```python
from build123d import *

# Parameters (mm, degrees)
F1_DEPTH = 135.89


with BuildPart() as f1:
    # F0 (on Front) → F1 (new body)
    with BuildSketch(Plane.XZ):
        with BuildLine():
            ThreePointArc((-0.402361, -59.350092), (-14.92337, -57.568817), (-28.607244, -52.393469))
            ThreePointArc((-28.607244, -52.393469), (-56.848471, -62.044811), (-86.337414, -57.449427))
            ThreePointArc((-86.337414, -57.449427), (-61.850793, -119.454468), (-0.402361, -145.306161))
            ThreePointArc((-0.402361, -145.306161), (20.97924, -102.328126), (-0.402361, -59.350092))
        make_face()
        with BuildLine():
            ThreePointArc((5.353071, 26.413075), (1.351735, 13.475031), (0, 0))
            ThreePointArc((0, 0), (26.5136, -53.799627), (85.330052, -65.546792))
            ThreePointArc((85.330052, -65.546792), (121.639734, -41.326507), (135.680214, 0))
            ThreePointArc((135.680214, 0), (99.219052, 60.146836), (29.028204, 55.640959))
            ThreePointArc((29.028204, 55.640959), (15.124492, 42.700633), (5.353071, 26.413075))
        make_face()
        with BuildLine():
            ThreePointArc((-31.83483, 54.332647), (-16.674524, 42.414806), (-5.886424, 26.430855))
            ThreePointArc((-5.886424, 26.430855), (-0.266385, 26.605869), (5.353071, 26.413075))
            ThreePointArc((5.353071, 26.413075), (15.124492, 42.700633), (29.028204, 55.640959))
            ThreePointArc((29.028204, 55.640959), (-1.577442, 63.087342), (-31.83483, 54.332647))
        make_face()
        with BuildLine():
            ThreePointArc((-28.607244, -52.393469), (-7.617664, -29.84732), (0, 0))
            ThreePointArc((0, 0), (-1.489415, 13.539203), (-5.886424, 26.430855))
            ThreePointArc((-5.886424, 26.430855), (-16.674524, 42.414806), (-31.83483, 54.332647))
            ThreePointArc((-31.83483, 54.332647), (-118.264652, 27.295814), (-86.337414, -57.449427))
            ThreePointArc((-86.337414, -57.449427), (-56.848471, -62.044811), (-28.607244, -52.393469))
        make_face()
        with BuildLine():
            ThreePointArc((85.330052, -65.546792), (26.5136, -53.799627), (0, 0))
            ThreePointArc((0, 0), (-7.617664, -29.84732), (-28.607244, -52.393469))
            ThreePointArc((-28.607244, -52.393469), (-14.92337, -57.568817), (-0.402361, -59.350092))
            ThreePointArc((-0.402361, -59.350092), (20.97924, -102.328126), (-0.402361, -145.306161))
            ThreePointArc((-0.402361, -145.306161), (58.145917, -122.282952), (85.330052, -65.546792))
        make_face()
        with BuildLine():
            ThreePointArc((-5.886424, 26.430855), (-1.489415, 13.539203), (0, 0))
            ThreePointArc((0, 0), (1.351735, 13.475031), (5.353071, 26.413075))
            ThreePointArc((5.353071, 26.413075), (-0.266385, 26.605869), (-5.886424, 26.430855))
        make_face()
    extrude(amount=F1_DEPTH)


solid = f1.part
```
Work out the finished part from the listing and answer in its coordinate system (mm). Give positions to 0.01 mm unless a question says otherwise; leave off trailing zeros. Order: outer loops, then holes, each group sorted by start corner. A loop starts at its lowest first (then second) coordinate and runs counter-clockwise, first axis right, second up.
1. Each of these flat-tipped pins is pushed along its axis until it touches: P1, Ø3, axis at y = -47, z = -43.5, coming from the +X side; P2, Ø8, axis at y = -48, z = 13.5, coming from the +X side; P3, Ø1, axis at y = -113.5, z = -109.5, coming from the -X side. Where does it stop, or does it pass through?
Result sheet:
P1: stops at x = 121.12
P2: stops at x = 135.01
P3: stops at x = -70.57
2. The mould has two halves that part along X. Classify faces 1 (the cylindrical face through (-1.132, -66.994, 63.095)), 2 (the flat face through (4, 0, -14)): released by +X, released by -X, zero draft, split by the parting line, or undercut.
Result sheet:
face 1: undercut
face 2: zero draft
3. Section B-B, the plane y = -48.5 is taken. Determine the outline of the cut face in (x, z), and give its area (3 significant figures).
Result sheet:
outline: (-86.34, -57.45) arc R85.96 ccw to (85.33, -65.55) arc R67.84 ccw to (135.68, 0) arc R67.84 ccw to (29.03, 55.64) arc R61.23 ccw to (-31.83, 54.33) arc R62.28 ccw (long way) to start
area: 40,500 mm2
4. Section A-A, the plane x = -37 is taken. Determine the outline of the cut face in (y, z), and give its area (3 significant figures).
Result sheet:
outline: (-135.89, -137.13) - (0, -137.13) - (0, 56.92) - (-135.89, 56.92) - close
area: 26,400 mm2
5. Section C-C, the plane z = 40 is taken. Determine the outline of the cut face in (x, y).
Result sheet:
outline: (-110.02, -135.89) - (122.63, -135.89) - (122.63, 0) - (-110.02, 0) - close
6. Straight lines are drawn through the part: L1, parallel to Z at x = 1, y = -96; L2, parallel to X at y = -113, z = 25.5; L3, parallel to Z at x = -68, y = -64. For each, find the intervals that lie inside material, in ascending order.
Result sheet:
L1: z = -145.29 to 63.09
L2: x = -119.11 to 130.71
L3: z = -112.44 to 62.02
